Geometry check sheet. Reference: the model listing, model coordinates, mm. Face numbers are marked on the shaded views. A direction names the side the tool comes from. Coordinates: 2 decimals unless noted, no trailing zeros. Write each loop counter-clockwise with the first axis right and the second up, starting at its lowest first coordinate (ties: lowest second). Pieces come first, ordered by that corner, then holes. Notation, with made-up numbers: (39, 80.5) -> (89, 80.5) arc R9 cw to (89, 92.5) -> close; hole circle Ø1 at (58.25, -2). An arc over 180 degrees is marked (long way). Answer in a Markdown table with one row per item. Add a question column.
Q1. Release check for a two-part mould opening along Z. For the marked faces 1, 2 and 3 record: pulls with the +Z half, pulls with the -Z half, needs draft (parallel to the pull), parting line crosses it, or undercut.
Q2. Tool access check on the marked faces 4 and 5. Record the directions out of +Z, -Z, +X, -X, +Y, -Y that give a thin tool (end or side, any length) a straight path to the whole face; none if there is none.
Q3. Thickness scan on line 1 (X direction, y = 1.75, z = 1.75); line 2 (Z direction, x = 4, y = -0.25); line 3 (Z direction, x = 3, y = -1.5). Record the ranges inside material, lowest first.
Q4. Gauge pin test, flat ends, axial feed: P1, Ø1.5, axis at y = 2, z = 1, coming from the +X side; P2, Ø1.1, axis at x = 0.5, y = -1.5, coming from the +Z side; P3, Ø0.8, axis at x = 0.5, z = 1.5, coming from the -Y side. Record the tip position at first contact, or that the pin passes through.
Q5. Section check A-A, the plane x = 6.5. Record the boundary of the cut face in (y, z).
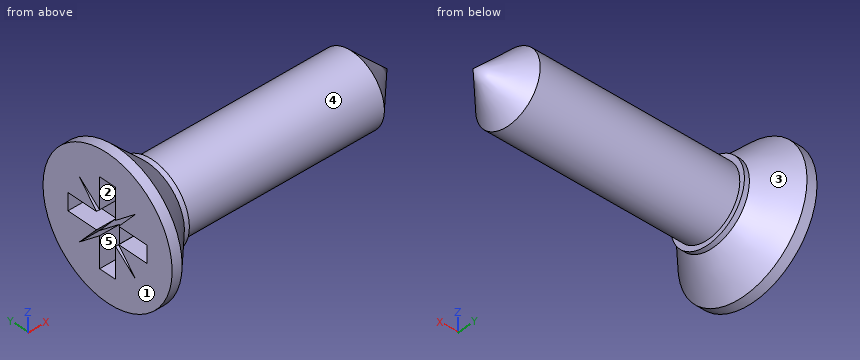
```python
from build123d import *

# Parameters (mm, degrees)
SKETCH2_R           = 1.75
BOSS_EXTRUDE1_DEPTH = 10
CUT_EXTRUDE1_DEPTH  = 1
DRAFT1_ANGLE        = -40
DRAFT2_ANGLE        = -40
DRAFT3_ANGLE        = -40
DRAFT4_ANGLE        = -40
DRAFT5_ANGLE        = -40
DRAFT6_ANGLE        = -40
DRAFT7_ANGLE        = -40
DRAFT8_ANGLE        = -40


with BuildPart() as part:
    # Sketch1 → Revolve1 (revolve)
    with BuildSketch(Plane(origin=(0, 0, 0), x_dir=(-1, 0, 0), z_dir=(0, 0, -1)), mode=Mode.PRIVATE) as revolve1_sk:
        Polygon((-2.25, 2), (-2.25, 0), (0, 0), (0, 3.5), (-0.5, 3.5), (-2, 2), align=None)
    revolve(revolve1_sk.sketch.rotate(Axis((2.25, 0, 0), (-1, 0, 0)), 270), axis=Axis((2.25, 0, 0), (-1, 0, 0)))

    # Sketch2 → Boss-Extrude1 (add)
    with BuildSketch(Plane(origin=(2.25, 0, 0), x_dir=(0, 0, -1), z_dir=(1, 0, 0))):
        Circle(SKETCH2_R)
    extrude(amount=BOSS_EXTRUDE1_DEPTH)

    # Sketch3 → Revolve2 (revolve)
    with BuildSketch(Plane.XY, mode=Mode.PRIVATE) as revolve2_sk:
        Polygon((12.25, 1.75), (12.25, 0), (14, 0), align=None)
    revolve(revolve2_sk.sketch.rotate(Axis((14.949975, 0, 0), (1, 0, 0)), 90), axis=Axis((14.949975, 0, 0), (1, 0, 0)))

    # Sketch4 → Cut-Extrude1 (cut)
    with BuildSketch(Plane.ZY):
        Polygon((-0.605426386, -0.43), (-0.605426386, -0.605426386), (-0.43, -0.605426386), (-0.43, -2.15), (0.43, -2.15), (0.43, -0.605426386), (0.605426386, -0.605426386), (0.605426386, -0.43), (2.15, -0.43), (2.15, 0.43), (0.605426386, 0.43), (0.605426386, 0.605426386), (0.43, 0.605426386), (0.43, 2.15), (-0.43, 2.15), (-0.43, 0.605426386), (-0.605426386, 0.605426386), (-0.605426386, 0.43), (-2.15, 0.43), (-2.15, -0.43), align=None)
    extrude(amount=-CUT_EXTRUDE1_DEPTH, mode=Mode.SUBTRACT)

    # Draft1
    draft1_faces = [part.faces().sort_by_distance(p)[0] for p in [
        (0.5, -0.605426386, -0.517713193),
    ]]
    draft(draft1_faces, Plane(origin=(1, -0.605426386, -0.43), x_dir=(0, 1, 0), z_dir=(0, 0, 1)), DRAFT1_ANGLE)

    # Draft2
    draft2_faces = [part.faces().sort_by_distance(p)[0] for p in [
        (0.5, -0.605426386, 0.517713193),
    ]]
    draft(draft2_faces, Plane(origin=(1, -2.15, 0.43), x_dir=(0, -1, 0), z_dir=(0, 0, -1)), DRAFT2_ANGLE)

    # Draft3
    draft3_faces = [part.faces().sort_by_distance(p)[0] for p in [
        (0.5, -0.591313301, 0.605426386),
    ]]
    draft(draft3_faces, Plane(origin=(1, -0.43, 0.605426386), x_dir=(0, 0, 1), z_dir=(0, 1, 0)), DRAFT3_ANGLE)

    # Draft4
    draft4_faces = [part.faces().sort_by_distance(p)[0] for p in [
        (0.5, 0.517713193, 0.605426386),
    ]]
    draft(draft4_faces, Plane(origin=(1, 0.43, 2.15), x_dir=(0, 0, -1), z_dir=(0, -1, 0)), DRAFT4_ANGLE)

    # Draft5
    draft5_faces = [part.faces().sort_by_distance(p)[0] for p in [
        (0.5, 0.605426386, 0.591313301),
    ]]
    draft(draft5_faces, Plane(origin=(1, 0.605426386, 0.43), x_dir=(0, -1, 0), z_dir=(0, 0, -1)), DRAFT5_ANGLE)

    # Draft6
    draft6_faces = [part.faces().sort_by_distance(p)[0] for p in [
        (0.5, 0.605426386, -0.517713193),
    ]]
    draft(draft6_faces, Plane(origin=(1, 2.15, -0.43), x_dir=(0, 1, 0), z_dir=(0, 0, 1)), DRAFT6_ANGLE)

    # Draft7
    draft7_faces = [part.faces().sort_by_distance(p)[0] for p in [
        (0.5, 0.591313301, -0.605426386),
    ]]
    draft(draft7_faces, Plane(origin=(1, 0.43, -0.605426386), x_dir=(0, 0, -1), z_dir=(0, -1, 0)), DRAFT7_ANGLE)

    # Draft8
    draft8_faces = [part.faces().sort_by_distance(p)[0] for p in [
        (0.5, -0.591313301, -0.605426386),
    ]]
    draft(draft8_faces, Plane(origin=(1, -0.43, -2.15), x_dir=(0, 0, 1), z_dir=(0, 1, 0)), DRAFT8_ANGLE)


solid = part.part
```
Calculated:
| question | item | result |
|---|---|---|
| 1 | face 1 | needs draft |
| 1 | face 2 | undercut |
| 1 | face 3 | parting line crosses it |
| 2 | face 4 | +X |
| 2 | face 5 | -X |
| 3 | line 1 | x = 0 to 1.53 |
| 3 | line 2 | z = -1.73 to 1.73 |
| 3 | line 3 | z = -0.9 to 0.9 |
| 4 | P1 | stops at x = 12.51 |
| 4 | P2 | stops at z = 3.37 |
| 4 | P3 | stops at y = -3.32 |
| 5 | outline | circle Ø3.5 at (0, 0) |
